from build123d import *

# Parameters (mm, degrees)
SKETCH1_R           = 10.9982
SKETCH1_R_2         = 1.397
BOSS_EXTRUDE1_DEPTH = 12.7
SKETCH2_W           = 4.603016963
SKETCH2_H           = 14.605
BOSS_EXTRUDE2_DEPTH = 2.54


with BuildPart() as part:
    # Sketch1 → Boss-Extrude1 (new body)
    with BuildSketch(Plane(origin=(0, 0, 0), x_dir=(1, 0, 0), z_dir=(0, 1, 0))):
        with Locations(Location((0, 0, 0), (0, 0, 270))):
            Circle(SKETCH1_R)
        with Locations(Location((3.7211, 6.44513426, 0), (0, 0, 270))):
            Circle(SKETCH1_R_2, mode=Mode.SUBTRACT)
        with Locations(Location((-3.7211, -6.44513426, 0), (0, 0, 270))):
            Circle(SKETCH1_R_2, mode=Mode.SUBTRACT)
    extrude(amount=BOSS_EXTRUDE1_DEPTH)

    # Sketch2 → Boss-Extrude2 (add)
    with BuildSketch(Plane(origin=(0, 12.7, 0), x_dir=(1, 0, 0), z_dir=(0, 1, 0))):
        with Locations((10.525491519, 0)):
            Rectangle(SKETCH2_W, SKETCH2_H)
    extrude(amount=-BOSS_EXTRUDE2_DEPTH)


solid = part.part
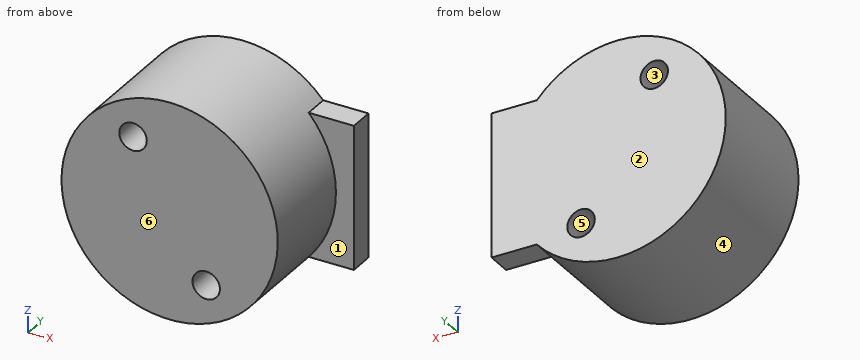
Work out the finished part from the listing and answer in its coordinate system (mm). Face numbers are marked on the shaded views. A direction names the side the tool comes from. Give positions to 0.01 mm unless a question says otherwise; leave off trailing zeros. Write each loop counter-clockwise with the first axis right and the second up, starting at its lowest first coordinate (ties: lowest second). Pieces come first, ordered by that corner, then holes.
Q1. A tool of negligible diameter and unlimited length cuts with its end or side. For the marked faces 1 and 2, from which of +Z, -Z, +X, -X, +Y, -Y can it reach the whole face along a straight path? Write none if from no direction.
Answer:
face 1: +X, -Y
face 2: +Z, -Z, +X, -X, +Y
Q2. Straight lines are drawn through the part: L1, parallel to Z at x = 9.25, y = 11.5; L2, parallel to X at y = 0.5, z = -7.25; L3, parallel to Z at x = -5, y = 11.5. For each, find the intervals that lie inside material, in ascending order.
Answer:
L1: z = -7.3 to 7.3
L2: x = -8.27 to 2.58, 4.86 to 8.27
L3: z = -9.8 to 5.88, 7.01 to 9.8
Q3. Given pin 1 (2 mm diameter, centred on y = 2.5, z = -3, fed in from -X); pin 2 (2 mm diameter, centred on x = 3.72, z = -6.45, fed in from +Y); pin 3 (6 mm diameter, centred on x = 5.5, y = 10.5, fed in from +Z); pin 4 (2 mm diameter, centred on x = 11, y = 12, fed in from -Z), each flat-ended and moving along its own axis, determine where each tip first touches the part or whether it passes through.
Answer:
pin 1: stops at x = -10.81
pin 2: passes through
pin 3: stops at z = 10.71
pin 4: stops at z = -7.3
Q4. The part is cut by section A-A on x = -2.75. Give the vertices of the cut face in (y, z), and give its area (3 significant figures).
Answer:
outline: (0, -10.65) - (12.7, -10.65) - (12.7, 5.44) - (0, 5.44) - close; (0, 7.45) - (12.7, 7.45) - (12.7, 10.65) - (0, 10.65) - close
area: 245 mm2
Q5. For a pull along X with two mould halves and no side action, classify the marked faces 3, 4, 5 and 6 as released by +X, released by -X, zero draft, split by the parting line, or undercut.
Answer:
face 3: undercut
face 4: split by the parting line
face 5: undercut
face 6: zero draft
Q6. The part is cut by section B-B on x = 10. Give the vertices of the cut face in (y, z), and give its area (3 significant figures).
Answer:
outline: (0, -4.58) - (10.16, -4.58) - (10.16, -7.3) - (12.7, -7.3) - (12.7, 7.3) - (10.16, 7.3) - (10.16, 4.58) - (0, 4.58) - close
area: 130 mm2
Q7. The part is cut by section D-D on y = 2. Give the vertices of the cut face in (x, z).
Answer:
outline: circle Ø22 at (0, 0); hole circle Ø2.79 at (-3.72, 6.45); hole circle Ø2.79 at (3.72, -6.45)
Q8. The part is cut by section C-C on z = 0. Give the vertices of the cut face in (x, y), and give its area (3 significant figures).
Answer:
outline: (-11, 0) - (11, 0) - (11, 10.16) - (12.83, 10.16) - (12.83, 12.7) - (-11, 12.7) - close
area: 284 mm2
